The drawing under review shows one solid part. Ordinate dimensions are in mm from its lowest x, y, z. A direction names the side the tool comes from. Give positions to 0.01 mm unless a question says otherwise; leave off trailing zeros. Order: outer loops, then holes, each group sorted by start corner. A loop starts at its lowest first (then second) coordinate and runs counter-clockwise, first axis right, second up. Notation, with made-up numbers: (83, 70) - (126, 70) arc R36 cw to (126, 105) - close; hole circle Ø8 at (36.25, -35.75). An arc over 180 degrees is marked (long way). Write item = value, one per line. Start each with the question number.
1. Wall thickness on probe 1 along X at (y, z) = (35.95, 9.65); probe 2 along Z at (x, y) = (30, 10.5); probe 3 along Z at (x, y) = (24.5, 27.5): over which ranges is each line inside the solid? List them lowest first.
2. We need section C-C, the plane y = 30. Give the boundary of the cut face in (x, z).
3. We need section A-A, the plane x = 18.65. Give the boundary of the cut face in (y, z).
4. Mouldability with a two-part tool opening along Y and no side actions: class the marked faces 3, 4, 5 and 6 as pulls with the +Y half, pulls with the -Y half, needs draft (parallel to the pull), parting line crosses it, or undercut.
5. For P1, Ø2, axis at y = 19.5, z = 11.5, coming from the +X side (1 decimal); P2, Ø8, axis at y = 11, z = 5, coming from the +X side; P3, Ø1.5, axis at x = 30, y = 14.5, coming from the +Z side, all flat-tipped, find the tip position at first contact; note any pin that passes through.
6. We need section D-D, the plane x = 7.5. Give the boundary of the cut face in (y, z).
7. We need section B-B, the plane z = 10.5. Give the boundary of the cut face in (x, y).
8. Machinability: for the marked faces 1 and 2, which of the approach directions +Z, -Z, +X, -X, +Y, -Y give a long, thin tool a straight path to every point of the face, cutting with its end or side? Answer none if there is none.
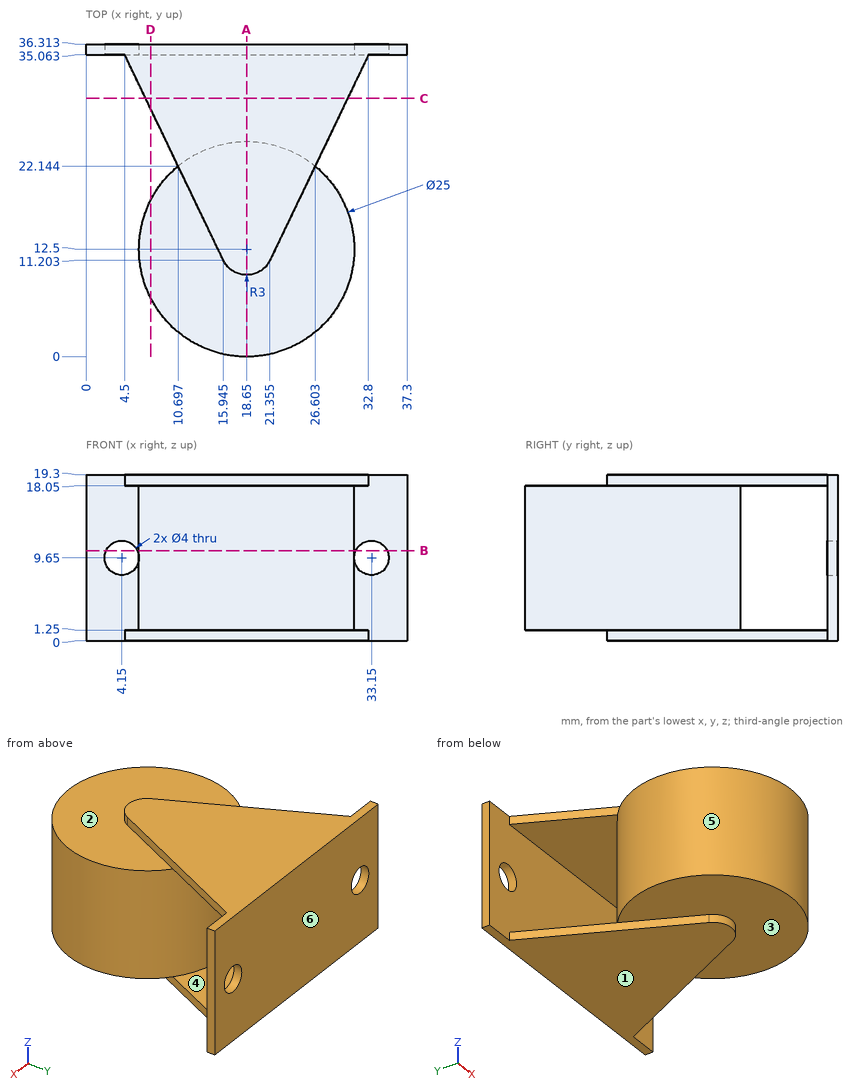
Model answer:
q1.probe_1 = 0 to 2.15, 6.15 to 31.15, 35.15 to 37.3
q1.probe_2 = 1.25 to 18.05
q1.probe_3 = 0 to 1.25, 18.05 to 19.3
q2.outline = (6.93, 0) - (30.37, 0) - (30.37, 1.25) - (6.93, 1.25) - close; (6.93, 18.05) - (30.37, 18.05) - (30.37, 19.3) - (6.93, 19.3) - close
q3.outline = (0, 1.25) - (9.5, 1.25) - (9.5, 0) - (36.31, 0) - (36.31, 19.3) - (9.5, 19.3) - (9.5, 18.05) - (0, 18.05) - close; hole (25, 1.25) - (35.06, 1.25) - (35.06, 18.05) - (25, 18.05) - close
q4.face_3 = needs draft
q4.face_4 = undercut
q4.face_5 = undercut
q4.face_6 = pulls with the +Y half
q5.P1 = 29.6
q5.P2 = 31.15
q5.P3 = 18.05
q6.outline = (6.85, 1.25) - (18.15, 1.25) - (18.15, 18.05) - (6.85, 18.05) - close; (28.81, 0) - (36.31, 0) - (36.31, 19.3) - (28.81, 19.3) - (28.81, 18.05) - (35.06, 18.05) - (35.06, 1.25) - (28.81, 1.25) - close
q7.outline = (0, 35.06) - (2.34, 35.06) - (2.34, 36.31) - (0, 36.31) - close; (5.96, 35.06) - (31.34, 35.06) - (31.34, 36.31) - (5.96, 36.31) - close; circle Ø25 at (18.65, 12.5); (34.96, 35.06) - (37.3, 35.06) - (37.3, 36.31) - (34.96, 36.31) - close
q8.face_1 = -Z, +X, -X, +Y, -Y
q8.face_2 = +Z, -Y
